Source: three-view drawing plus pictorial views. Frame: mm from the lowest corner of the part. A direction names the side the tool comes from. Round coordinates to 2 decimals unless told otherwise and drop trailing zeros. Write each loop counter-clockwise with the first axis right and the second up, starting at its lowest first coordinate (ties: lowest second). Pieces come first, ordered by that corner, then holes. Notation, with made-up numbers: M 88,62 L 121,62 A9 ccw 121,67 Z; hole C 15,-4 d1. An arc over 180 degrees is marked long. Put each result on its own line as item: value. Start each with the question number.
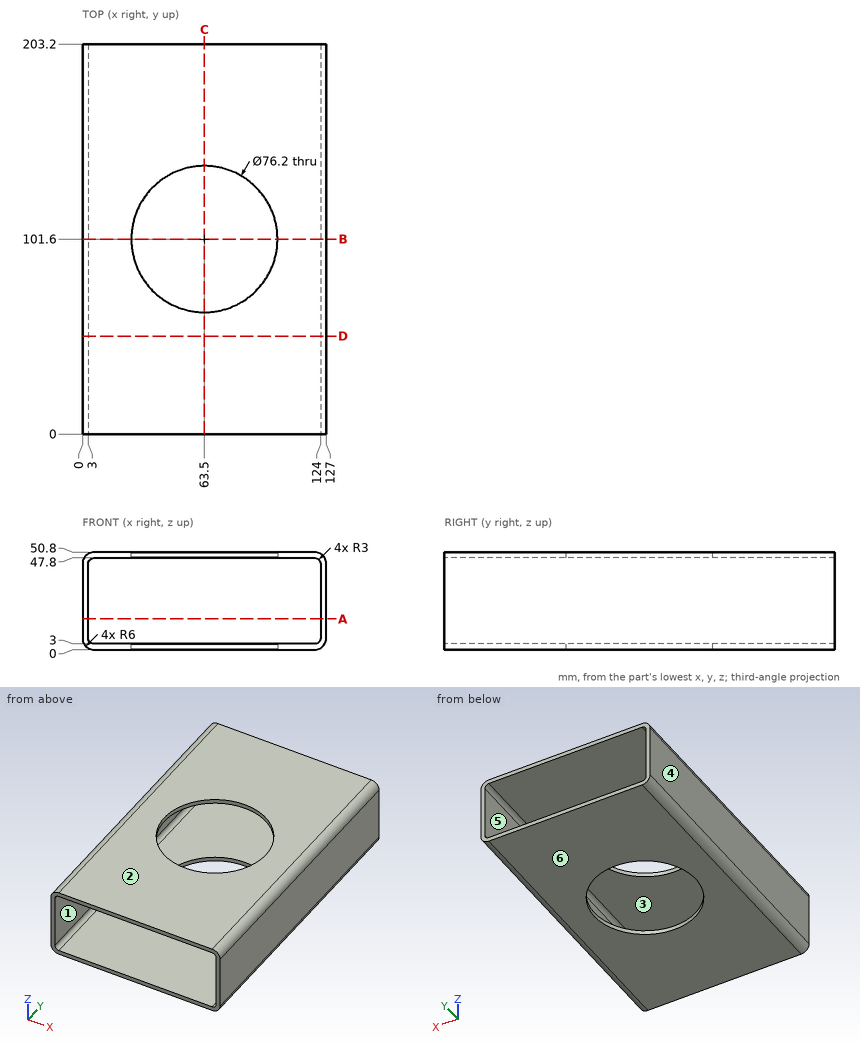
(1) Section query D-D (y = 51). Return loops of the section in (x, z), and give its area (3 significant figures).
(2) Section query B-B (y = 101.6). Return loops of the section in (x, z), and give its area (3 significant figures).
(3) Section query A-A (z = 16). Return loops of the section in (x, y).
(4) Pull-direction query (X, two-part tool) for the marked faces 1, 2, 3 and 4; classes: +X half, -X half, draft (parallel to the pull), parting line (faces both ways), or undercut.
(5) Ray query, line 1 along Z through (x, y) = (34.5, 64.5); line 2 along X through (y, z) = (182.5, 42.5); line 3 along Y through (x, z) = (63.5, 1.85). Return the intervals inside material, ascending.
(6) Section query C-C (x = 63.5). Return loops of the section in (y, z).
(7) Access query for the marked faces 5 and 6. Directions: +Z, -Z, +X, -X, +Y, -Y. A direction counts if a zero-diameter tool reaches every point of the face in a straight line with its end or side. Return the directions, or none.
Entries:
1. outline: M 0,6 A6 ccw 6,0 L 121,0 A6 ccw 127,6 L 127,44.8 A6 ccw 121,50.8 L 6,50.8 A6 ccw 0,44.8 Z; hole M 3,6 A3 ccw 6,3 L 121,3 A3 ccw 124,6 L 124,44.8 A3 ccw 121,47.8 L 6,47.8 A3 ccw 3,44.8 Z
1. area: 1,010 mm2
2. outline: M 0,6 A6 ccw 6,0 L 25.4,0 L 25.4,3 L 6,3 A3 cw 3,6 L 3,44.8 A3 cw 6,47.8 L 25.4,47.8 L 25.4,50.8 L 6,50.8 A6 ccw 0,44.8 Z; M 101.6,0 L 121,0 A6 ccw 127,6 L 127,44.8 A6 ccw 121,50.8 L 101.6,50.8 L 101.6,47.8 L 121,47.8 A3 cw 124,44.8 L 124,6 A3 cw 121,3 L 101.6,3 Z
2. area: 550 mm2
3. outline: M 0,0 L 3,0 L 3,203.2 L 0,203.2 Z; M 124,0 L 127,0 L 127,203.2 L 124,203.2 Z
4. face 1: undercut
4. face 2: draft
4. face 3: undercut
4. face 4: -X half
5. line 1: 0 to 3, 47.8 to 50.8
5. line 2: 0 to 3, 124 to 127
5. line 3: 0 to 63.5, 139.7 to 203.2
6. outline: M 0,0 L 63.5,0 L 63.5,3 L 0,3 Z; M 0,47.8 L 63.5,47.8 L 63.5,50.8 L 0,50.8 Z; M 139.7,0 L 203.2,0 L 203.2,3 L 139.7,3 Z; M 139.7,47.8 L 203.2,47.8 L 203.2,50.8 L 139.7,50.8 Z
7. face 5: +Y, -Y
7. face 6: -Z, +X, -X, +Y, -Y
